from build123d import *

# Parameters (mm, degrees)
CYLINDER004_R     = 1.5
CYLINDER004_DEPTH = 10
CYLINDER003_R     = 1.5
CYLINDER003_DEPTH = 10
CYLINDER002_R     = 1.5
CYLINDER002_DEPTH = 10
CYLINDER001_R     = 1.5
CYLINDER001_DEPTH = 10
CYLINDER_R        = 1.5
CYLINDER_DEPTH    = 10
BOX_W             = 50
BOX_H             = 10
BOX_DEPTH         = 3


with BuildPart() as cilindro004:
    # Cylinder004 → Cylinder004 (new body)
    with BuildSketch(Plane(origin=(45, 5, -1), x_dir=(1, 0, 0), z_dir=(0, 0, 1))):
        Circle(CYLINDER004_R)
    extrude(amount=CYLINDER004_DEPTH)


with BuildPart() as cilindro003:
    # Cylinder003 → Cylinder003 (new body)
    with BuildSketch(Plane(origin=(35, 5, -1), x_dir=(1, 0, 0), z_dir=(0, 0, 1))):
        Circle(CYLINDER003_R)
    extrude(amount=CYLINDER003_DEPTH)


with BuildPart() as cilindro002:
    # Cylinder002 → Cylinder002 (new body)
    with BuildSketch(Plane(origin=(25, 5, -1), x_dir=(1, 0, 0), z_dir=(0, 0, 1))):
        Circle(CYLINDER002_R)
    extrude(amount=CYLINDER002_DEPTH)


with BuildPart() as cilindro001:
    # Cylinder001 → Cylinder001 (new body)
    with BuildSketch(Plane(origin=(15, 5, -1), x_dir=(1, 0, 0), z_dir=(0, 0, 1))):
        Circle(CYLINDER001_R)
    extrude(amount=CYLINDER001_DEPTH)


with BuildPart() as cilindro:
    # Cylinder → Cylinder (new body)
    with BuildSketch(Plane(origin=(5, 5, -1), x_dir=(1, 0, 0), z_dir=(0, 0, 1))):
        Circle(CYLINDER_R)
    extrude(amount=CYLINDER_DEPTH)


with BuildPart() as cut004:
    # Box → Box (new body)
    with BuildSketch(Plane.XY):
        with Locations((25, 5)):
            Rectangle(BOX_W, BOX_H)
    extrude(amount=BOX_DEPTH)

    # Cut: cut Cilindro
    add(cilindro.part, mode=Mode.SUBTRACT)

    # Cut001: cut Cilindro001
    add(cilindro001.part, mode=Mode.SUBTRACT)

    # Cut002: cut Cilindro002
    add(cilindro002.part, mode=Mode.SUBTRACT)

    # Cut003: cut Cilindro003
    add(cilindro003.part, mode=Mode.SUBTRACT)

    # Cut004: cut Cilindro004
    add(cilindro004.part, mode=Mode.SUBTRACT)


solid = cut004.part
Input: part model. Units: mm. Frame: model coordinates. Coordinates: 2 decimals unless noted, no trailing zeros. Loops run counter-clockwise (first coordinate to the right, second up) from the corner with the lowest first, then second, coordinate; pieces in that order, holes last.
(1) Material intervals for probe 1 along X at (y, z) = (5, 2.35); probe 2 along Y at (x, z) = (25, 1.95); probe 3 along X at (y, z) = (6, 0.25), sorted ascending.
(2) Pull-direction query (X, two-part tool) for faces 1 (the face through (50, 5, 1)), 2 (the face through (25, 7, 3)), 3 (the face through (23.5, 5.07, 1.48)); classes: released by +X, released by -X, zero draft, split by the parting line, or undercut.
(3) First-contact query: pin 1 Ø3.5 at (x, y) = (25, 5) entering from -Z; pin 2 Ø2.5 at (x, y) = (15, 5) entering from -Z (3 decimals). Flat tips, straight axial feed; report the tip coordinate or a pass-through.
(4) Section B-B on x = 15. Return the cut outline in (y, z), then the cut area to 3 significant figures.
(5) Section D-D on x = 35.5. Return the cut outline in (y, z), then the cut area to 3 significant figures.
(6) Section C-C on y = 4.5. Return the cut outline in (x, z), then the cut area to 3 significant figures.
(7) Section A-A on z = 1.3. Return the cut outline in (x, y).
Data:
1. probe 1: x = 0 to 3.5, 6.5 to 13.5, 16.5 to 23.5, 26.5 to 33.5, 36.5 to 43.5, 46.5 to 50
1. probe 2: y = 0 to 3.5, 6.5 to 10
1. probe 3: x = 0 to 3.88, 6.12 to 13.88, 16.12 to 23.88, 26.12 to 33.88, 36.12 to 43.88, 46.12 to 50
2. face 1: released by +X
2. face 2: zero draft
2. face 3: undercut
3. pin 1: stops at z = 0
3. pin 2: passes through
4. outline: (0, 0) - (3.5, 0) - (3.5, 3) - (0, 3) - close; (6.5, 0) - (10, 0) - (10, 3) - (6.5, 3) - close
4. area: 21.0 mm2
5. outline: (0, 0) - (3.59, 0) - (3.59, 3) - (0, 3) - close; (6.41, 0) - (10, 0) - (10, 3) - (6.41, 3) - close
5. area: 21.5 mm2
6. outline: (0, 0) - (3.59, 0) - (3.59, 3) - (0, 3) - close; (6.41, 0) - (13.59, 0) - (13.59, 3) - (6.41, 3) - close; (16.41, 0) - (23.59, 0) - (23.59, 3) - (16.41, 3) - close; (26.41, 0) - (33.59, 0) - (33.59, 3) - (26.41, 3) - close; (36.41, 0) - (43.59, 0) - (43.59, 3) - (36.41, 3) - close; (46.41, 0) - (50, 0) - (50, 3) - (46.41, 3) - close
6. area: 108 mm2
7. outline: (0, 0) - (50, 0) - (50, 10) - (0, 10) - close; hole circle Ø3 at (5, 5); hole circle Ø3 at (15, 5); hole circle Ø3 at (25, 5); hole circle Ø3 at (35, 5); hole circle Ø3 at (45, 5)
